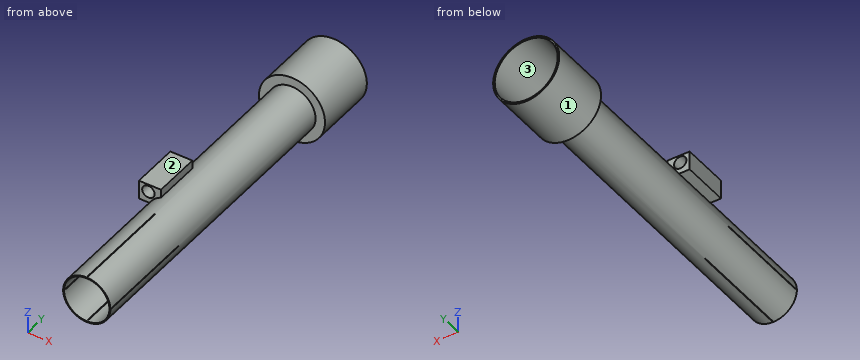
```python
from build123d import *

# Parameters (mm, degrees)
SKETCH1_R           = 9.525
BOSS_EXTRUDE1_DEPTH = 150
SKETCH2_R           = 9.144
CUT_EXTRUDE1_DEPTH  = 177.8
CUT_EXTRUDE3_START  = 10.16
SKETCH3_W           = 0.254
SKETCH3_H           = 40.64
CUT_EXTRUDE3_DEPTH  = 1.27
CIRPATTERN1_COUNT   = 4
SKETCH9_R           = 13.335
BOSS_EXTRUDE2_DEPTH = 25.4
SKETCH10_R          = 12.7
CUT_EXTRUDE5_DEPTH  = 24.13
CUT_EXTRUDE6_START  = -24.13
SKETCH11_R          = 9.144
CUT_EXTRUDE6_DEPTH  = 24.13
BOSS_EXTRUDE3_START = 50.8
SKETCH12_W          = 8.89
SKETCH12_H          = 7.62
BOSS_EXTRUDE3_DEPTH = 19.05
SKETCH13_R          = 2.5
CUT_EXTRUDE7_DEPTH  = 19.05
CUT_EXTRUDE8_START  = 60.96
SKETCH14_R          = 9.144
CUT_EXTRUDE8_DEPTH  = 60.96


with BuildPart() as part:
    # Sketch1 → Boss-Extrude1 (new body)
    with BuildSketch(Plane(origin=(0, 0, 0), x_dir=(1, 0, 0), z_dir=(0, 1, 0))):
        with Locations(Location((0, 0, 0), (0, 0, 270))):
            Circle(SKETCH1_R)
    extrude(amount=BOSS_EXTRUDE1_DEPTH)

    # Sketch2 → Cut-Extrude1 (cut)
    with BuildSketch(Plane(origin=(0, 150, 0), x_dir=(1, 0, 0), z_dir=(0, 1, 0))):
        with Locations(Location((0, 0, 0), (0, 0, 270))):
            Circle(SKETCH2_R)
    extrude(amount=-CUT_EXTRUDE1_DEPTH, mode=Mode.SUBTRACT)

    # Sketch3 → Cut-Extrude3 (cut)
    with BuildSketch(Plane(origin=(0, 0, 0), x_dir=(0, 0, -1), z_dir=(1, 0, 0)).offset(CUT_EXTRUDE3_START)):
        with Locations((0, 21.082)):
            Rectangle(SKETCH3_W, SKETCH3_H)
    cut_extrude3 = extrude(amount=-CUT_EXTRUDE3_DEPTH, mode=Mode.SUBTRACT)

    # CirPattern1: Cut-Extrude3 ×4 about axis
    cirpattern1_axis = Axis((0, 0, 0), (0, 1, 0))
    for i in range(1, CIRPATTERN1_COUNT):
        add(cut_extrude3.rotate(cirpattern1_axis, i * 360 / CIRPATTERN1_COUNT), mode=Mode.SUBTRACT)

    # Sketch9 → Boss-Extrude2 (add)
    with BuildSketch(Plane(origin=(0, 150, 0), x_dir=(1, 0, 0), z_dir=(0, 1, 0))):
        with Locations(Location((0, 0, 0), (0, 0, 270))):
            Circle(SKETCH9_R)
    extrude(amount=-BOSS_EXTRUDE2_DEPTH)

    # Sketch10 → Cut-Extrude5 (cut)
    with BuildSketch(Plane(origin=(0, 150, 0), x_dir=(1, 0, 0), z_dir=(0, 1, 0))):
        with Locations(Location((0, 0, 0), (0, 0, 270))):
            Circle(SKETCH10_R)
    extrude(amount=-CUT_EXTRUDE5_DEPTH, mode=Mode.SUBTRACT)

    # Sketch11 → Cut-Extrude6 (cut)
    with BuildSketch(Plane.XZ.offset(-124.6).offset(CUT_EXTRUDE6_START)):
        with Locations(Location((0, 0, 0), (0, 0, 90))):
            Circle(SKETCH11_R)
    extrude(amount=CUT_EXTRUDE6_DEPTH, mode=Mode.SUBTRACT)

    # Sketch12 → Boss-Extrude3 (add)
    with BuildSketch(Plane(origin=(0, 0, 0), x_dir=(1, 0, 0), z_dir=(0, 1, 0)).offset(BOSS_EXTRUDE3_START)):
        with Locations((-8.255, -8.305027858)):
            Rectangle(SKETCH12_W, SKETCH12_H)
    extrude(amount=BOSS_EXTRUDE3_DEPTH)

    # Sketch13 → Cut-Extrude7 (cut)
    with BuildSketch(Plane(origin=(0, 69.85, 0), x_dir=(1, 0, 0), z_dir=(0, 1, 0))):
        with Locations(Location((-8.89, -9.067027858, 0), (0, 0, 270))):
            Circle(SKETCH13_R)
    extrude(amount=-CUT_EXTRUDE7_DEPTH, mode=Mode.SUBTRACT)

    # Sketch14 → Cut-Extrude8 (cut)
    with BuildSketch(Plane(origin=(0, 0, 0), x_dir=(1, 0, 0), z_dir=(0, 1, 0)).offset(CUT_EXTRUDE8_START)):
        with Locations(Location((0, 0, 0), (0, 0, 270))):
            Circle(SKETCH14_R)
    extrude(amount=-CUT_EXTRUDE8_DEPTH, mode=Mode.SUBTRACT)


solid = part.part
```
Build history of the part. All positions in model axes, mm. Face numbers are marked on the shaded views. Coordinates: 2 decimals unless noted, no trailing zeros. Write each loop counter-clockwise with the first axis right and the second up, starting at its lowest first coordinate (ties: lowest second). Pieces come first, ordered by that corner, then holes.
1. Band-saw the part on A-A, the plane y = 18. Give the cut face in (x, z) (3 decimals), and give its area (3 significant figures).
Answer block:
outline: (-9.524, -0.127) arc R9.525 ccw to (-0.127, -9.524) - (-0.127, -9.143) arc R9.144 cw to (-9.143, -0.127) - close; (-9.524, 0.127) - (-9.143, 0.127) arc R9.144 cw to (-0.127, 9.143) - (-0.127, 9.524) arc R9.525 ccw to start; (0.127, -9.524) arc R9.525 ccw to (9.524, -0.127) - (9.143, -0.127) arc R9.144 cw to (0.127, -9.143) - close; (0.127, 9.143) arc R9.144 cw to (9.143, 0.127) - (9.524, 0.127) arc R9.525 ccw to (0.127, 9.524) - close
area: 22.0 mm2
2. Drop flat-ended pins along their axis: pin 1 (1.5 mm diameter, centred on y = 24, z = 0.5, fed in from +X); pin 2 (2 mm diameter, centred on y = 18.5, z = 3, fed in from +X); pin 3 (1.7 mm diameter, centred on y = 61, z = 11, fed in from +X). Give the stop position or say it passes through.
Answer block:
pin 1: stops at x = 9.52
pin 2: stops at x = 9.31
pin 3: stops at x = -3.81
3. Drill centre lines: probe 1 along X at (y, z) = (134, 0) (3 decimals); probe 2 along Z at (x, y) = (0, 102.5) (3 decimals); probe 3 along Y at (x, z) = (-11.5, 5.25). Where is each one in solid material? Low to high.
Answer block:
probe 1: x = -13.335 to -12.7, 12.7 to 13.335
probe 2: z = -9.525 to -9.144, 9.144 to 9.525
probe 3: y = 50.8 to 69.85, 124.6 to 125.87
4. Band-saw the part on D-D, the plane y = 47.5. Give the cut face in (x, z) (3 decimals), and give its area (3 significant figures).
Answer block:
outline: circle Ø19.05 at (0, 0); hole circle Ø18.288 at (0, 0)
area: 22.3 mm2
5. Band-saw the part on C-C, the plane z = -1.5. Give the cut face in (x, y).
Answer block:
outline: (-13.25, 124.6) - (-9.41, 124.6) - (-9.41, 0) - (-9.02, 0) - (-9.02, 125.87) - (-12.61, 125.87) - (-12.61, 150) - (-13.25, 150) - close; (9.02, 0) - (9.41, 0) - (9.41, 124.6) - (13.25, 124.6) - (13.25, 150) - (12.61, 150) - (12.61, 125.87) - (9.02, 125.87) - close
6. Band-saw the part on B-B, the plane x = 4.5. Give the cut face in (y, z), and give its area (3 significant figures).
Answer block:
outline: (0, -8.39) - (124.6, -8.39) - (124.6, -12.55) - (150, -12.55) - (150, -11.88) - (125.87, -11.88) - (125.87, -7.96) - (0, -7.96) - close; (0, 7.96) - (125.87, 7.96) - (125.87, 11.88) - (150, 11.88) - (150, 12.55) - (124.6, 12.55) - (124.6, 8.39) - (0, 8.39) - close
area: 153 mm2
7. Pull direction X, two halves, no side cores. Call the marked faces 1, 2 and 3: released by +X, released by -X, zero draft, split by the parting line, or undercut.
Answer block:
face 1: split by the parting line
face 2: zero draft
face 3: undercut
